Source: CAD feature listing. Evaluate the final solid. Frame: model axes, mm. Face numbers are marked on the shaded views. Give positions to 0.01 mm unless a question says otherwise; leave off trailing zeros. Order: outer loops, then holes, each group sorted by start corner. A loop starts at its lowest first (then second) coordinate and runs counter-clockwise, first axis right, second up.
```python
from build123d import *

# Parameters (mm, degrees)
SKETCH1_W                      = 665
SKETCH1_H                      = 650
BOSS_EXTRUDE1_DEPTH            = 30
F_8_0_199_DIAMETER_HOLE1_D     = 5.0546
F_8_0_199_DIAMETER_HOLE1_DEPTH = 9.65
SKETCH4_W                      = 615
SKETCH4_H                      = 600
CUT_EXTRUDE1_DEPTH             = 20
SHELL_T                        = -2


with BuildPart() as part:
    # Sketch1 → Boss-Extrude1 (new body)
    with BuildSketch(Plane(origin=(0, 0, 0), x_dir=(1, 0, 0), z_dir=(0, 1, 0))):
        with Locations((332.5, 325)):
            Rectangle(SKETCH1_W, SKETCH1_H)
    extrude(amount=-BOSS_EXTRUDE1_DEPTH)

    # #8 (0.199) Diameter Hole1
    with Locations(Plane(origin=(0, 0, 0), x_dir=(1, 0, 0), z_dir=(0, 1, 0))):
        with Locations((68.25, 13.5), (13.5, 301), (596.75, 13.5), (651.5, 301), (651.5, 349), (596.75, 636.5), (68.25, 636.5), (13.5, 349)):
            Hole(F_8_0_199_DIAMETER_HOLE1_D / 2, depth=F_8_0_199_DIAMETER_HOLE1_DEPTH)

    # Sketch4 → Cut-Extrude1 (cut)
    with BuildSketch(Plane(origin=(0, 0, 0), x_dir=(1, 0, 0), z_dir=(0, 1, 0))):
        with Locations((332.5, 325)):
            Rectangle(SKETCH4_W, SKETCH4_H)
    extrude(amount=-CUT_EXTRUDE1_DEPTH, mode=Mode.SUBTRACT)

    # Shell
    shell_openings = [part.faces().sort_by_distance(p)[0] for p in [
        (25, -10, -325),
        (332.5, -10, -25),
        (640, -10, -325),
        (332.5, -10, -625),
        (332.5, -20, -325),
    ]]
    offset(amount=SHELL_T, openings=shell_openings, kind=Kind.INTERSECTION)


solid = part.part
```
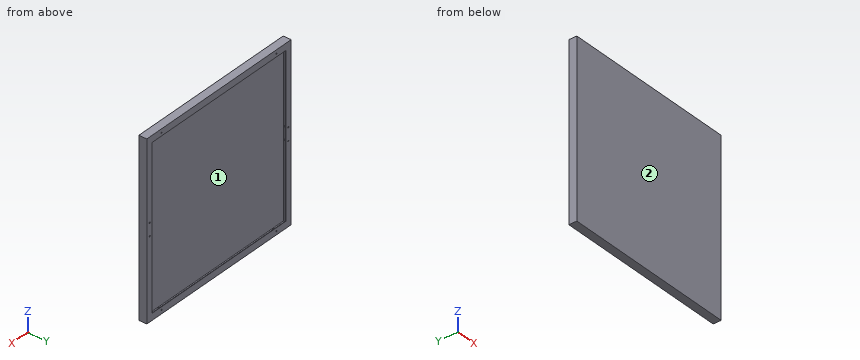
1) Pin query (flat end, axial travel): pin 1 (1.5 mm diameter, centred on x = 109, z = -235.5, fed in from +Y); pin 2 (3 mm diameter, centred on x = 596.75, z = -13.5, fed in from +Y). Return the tip coordinate at first contact, or that it passes through.
Report:
pin 1: stops at y = -28
pin 2: stops at y = -9.65
2) Material intervals for L1, parallel to X at y = -3, z = -301; L2, parallel to Z at x = 651.5, y = -6.5; L3, parallel to Z at x = 68.25, y = -3.75, sorted ascending.
Report:
L1: x = 0 to 2, 8.97 to 10.97, 16.03 to 18.03, 646.97 to 648.97, 654.03 to 656.03, 663 to 665
L2: z = -650 to -648, -353.53 to -351.53, -346.47 to -344.47, -305.53 to -303.53, -298.47 to -296.47, -2 to 0
L3: z = -650 to -648, -641.03 to -639.03, -633.97 to -631.97, -18.03 to -16.03, -10.97 to -8.97, -2 to 0
3) Section query B-B, the plane x = 109. Return the cut outline in (y, z).
Report:
outline: (-30, -650) - (0, -650) - (0, -625) - (-2, -625) - (-2, -648) - (-28, -648) - (-28, -2) - (-2, -2) - (-2, -25) - (0, -25) - (0, 0) - (-30, 0) - close
4) Section query A-A, the plane z = -316.5. Return the cut outline in (x, y), and give its area (3 significant figures).
Report:
outline: (0, -30) - (665, -30) - (665, 0) - (640, 0) - (640, -2) - (663, -2) - (663, -28) - (2, -28) - (2, -2) - (25, -2) - (25, 0) - (0, 0) - close
area: 1,530 mm2
5) Draft query along Z for the marked faces 1 and 2. Return one class per face: +Z half, -Z half, draft (parallel to the pull), parting line (faces both ways), or undercut.
Report:
face 1: undercut
face 2: draft
